```python
from build123d import *

# Parameters (mm, degrees)
PAD024_DEPTH         = 7.1
SKETCH051_W          = 7.4
SKETCH051_H          = 6.5
POCKET035_DEPTH      = 7.551
POCKET035_DEPTH_BACK = 7.551
SKETCH052_W          = 10
SKETCH052_H          = 7.5
POCKET036_DEPTH      = 19.501
POCKET036_DEPTH_BACK = 0.001
SKETCH053_R          = 0.75
POCKET037_DEPTH      = 16.25
CHAMFER007_SIZE      = 0.25
FILLET004_R          = 0.4
CHAMFER008_SIZE      = 0.25


with BuildPart() as part:
    # Sketch050 → Pad024 (new body)
    with BuildSketch(Plane.XZ.offset(3.55)):
        Polygon((5.5, -11.6), (5.5, -19.5), (-5.5, -19.5), (-5.5, -11.6), (-7.55, -11.6), (-7.55, -7), (7.55, -7), (7.55, -11.6), align=None)
    extrude(amount=PAD024_DEPTH)

    # Sketch051 → Pocket035 (cut, two sides)
    with BuildSketch(Plane.YZ) as pocket035_sk:
        with Locations((-3.7, -16.25)):
            Rectangle(SKETCH051_W, SKETCH051_H)
    extrude(amount=-POCKET035_DEPTH, mode=Mode.SUBTRACT)
    extrude(pocket035_sk.sketch, amount=POCKET035_DEPTH_BACK, mode=Mode.SUBTRACT)

    # Sketch052 → Pocket036 (cut, two sides)
    with BuildSketch(Plane.XY) as pocket036_sk:
        with Locations((0, -3.75)):
            Rectangle(SKETCH052_W, SKETCH052_H)
    extrude(amount=-POCKET036_DEPTH, mode=Mode.SUBTRACT)
    extrude(pocket036_sk.sketch, amount=POCKET036_DEPTH_BACK, mode=Mode.SUBTRACT)

    # Sketch053 → Pocket037 (cut, symmetric)
    with BuildSketch(Plane.XY):
        with Locations((0, -8.6)):
            Circle(SKETCH053_R)
        with Locations((2.9, -8.6)):
            Circle(SKETCH053_R)
        with Locations((-2.9, -8.6)):
            Circle(SKETCH053_R)
    extrude(amount=POCKET037_DEPTH, both=True, mode=Mode.SUBTRACT)

    # Chamfer007
    chamfer007_edges = [part.edges().sort_by_distance(p)[0] for p in [
        (2.15, -8.6, -7),
        (-0.75, -8.6, -7),
        (-3.65, -8.6, -7),
    ]]
    chamfer(chamfer007_edges, length=CHAMFER007_SIZE)

    # Fillet004
    fillet004_edges = [part.edges().sort_by_distance(p)[0] for p in [
        (-7.55, -7.1, -7),
        (7.55, -7.1, -7),
        (-7.55, -7.1, -11.6),
        (5.5, -9.025, -19.5),
        (-5.5, -9.025, -19.5),
        (7.55, -7.1, -11.6),
    ]]
    fillet(fillet004_edges, radius=FILLET004_R)

    # Chamfer008
    chamfer008_edges = [part.edges().sort_by_distance(p)[0] for p in [
        (0, -10.65, -7),
        (0, -10.65, -19.5),
        (-7.55, -3.55, -9.3),
        (7.55, -3.55, -9.3),
    ]]
    chamfer(chamfer008_edges, length=CHAMFER008_SIZE)


with BuildPart() as part_1:
    # Body011 placement: moved
    add(part.part.moved(Location((-18, 7.1, 0))))


solid = part_1.part
```
For this review, take the finished solid that the model builds, in its own axes (mm). A direction names the side the tool comes from. Give positions to 0.01 mm unless a question says otherwise; leave off trailing zeros. Write each loop counter-clockwise with the first axis right and the second up, starting at its lowest first coordinate (ties: lowest second). Pieces come first, ordered by that corner, then holes.
Item 1: Insertion check: P1, Ø0.6, axis at x = -23.5, y = 2.5, coming from the -Z side; P2, Ø0.9, axis at x = -15.1, y = -1.5, coming from the +Z side; P3, Ø0.8, axis at x = -18, y = -1, coming from the +Z side. Each pin has a flat end and moves straight along its axis. Give the tip position at first contact, or say it passes through.
Item 2: Take a section at B-B (y = 0.5). Give the boundary of the cut face in (x, z).
Item 3: The part is to be moulded in two halves that separate along X. For faces 1 (the face through (-25.55, 0, -9)), 2 (the face through (-18, -1, -16.25)), 3 (the face through (-24, 3.55, -9)), say which applies: +X half, -X half, draft (parallel to the pull), parting line (faces both ways), or undercut.
Item 4: Take a section at A-A (z = -14). Give the boundary of the cut face in (x, y), and give its area (3 significant figures).
Item 5: Wall thickness on probe 1 along Y at (x, z) = (-15.1, -9.5); probe 2 along X at (y, z) = (-1.25, -8); probe 3 along Y at (x, z) = (-20.5, -14.75): over which ranges is each line inside the solid? List them lowest first.
Item 6: Machinability: for faces 4 (the face through (-18, -0.4, -13)), 5 (the face through (-12, 0, -11.6)), 6 (the face through (-18.75, -1.47, -11.69)), which of the approach directions +Z, -Z, +X, -X, +Y, -Y give a long, thin tool a straight path to every point of the face, cutting with its end or side? Answer none if there is none.
Item 7: Take a section at C-C (x = -18). Give the boundary of the cut face in (y, z), and give its area (3 significant figures).
Established:
1. P1: stops at z = -13
1. P2: stops at z = -16.25
1. P3: stops at z = -7.1
2. outline: (-25.55, -11.2) arc R0.4 ccw to (-25.15, -11.6) - (-23.5, -11.6) - (-23.5, -13) - (-23, -13) - (-23, -7) - (-25.15, -7) arc R0.4 ccw to (-25.55, -7.4) - close; (-13, -13) - (-12.5, -13) - (-12.5, -11.6) - (-10.85, -11.6) arc R0.4 ccw to (-10.45, -11.2) - (-10.45, -7.4) arc R0.4 ccw to (-10.85, -7) - (-13, -7) - close
3. face 1: -X half
3. face 2: undercut
3. face 3: draft
4. outline: (-23.5, -3.3) - (-23.25, -3.55) - (-12.75, -3.55) - (-12.5, -3.3) - (-12.5, -0.3) - (-13, -0.3) - (-13, -0.4) - (-23, -0.4) - (-23, -0.3) - (-23.5, -0.3) - close; hole circle Ø1.5 at (-20.9, -1.5); hole circle Ø1.5 at (-18, -1.5); hole circle Ø1.5 at (-15.1, -1.5)
4. area: 29.4 mm2
5. probe 1: y = -3.55 to -2.25, -0.75 to -0.4
5. probe 2: x = -25.55 to -21.61, -20.19 to -18.71, -17.29 to -15.81, -14.39 to -10.45
5. probe 3: y = -3.55 to -2.13, -0.87 to -0.4
6. face 4: +Z, -Z, +Y
6. face 5: -Z, +X, +Y, -Y
6. face 6: +Z
7. outline: (-3.55, -19.25) - (-3.3, -19.5) - (-0.4, -19.5) - (-0.4, -7) - (-0.5, -7) - (-0.75, -7.25) - (-0.75, -16.25) - (-2.25, -16.25) - (-2.25, -7.25) - (-2.5, -7) - (-3.3, -7) - (-3.55, -7.25) - close
7. area: 25.4 mm2
